from build123d import *

# Parameters (mm, degrees)
F1_DEPTH  = 873.125
F4_DEPTH  = 12.7
F5_W      = 304.8
F5_H      = 171.45
F5_R      = 17.4625
F5_W_2    = 234.95
F6_DEPTH  = 25.4
F7_W      = 101.6
F7_H      = 787.4
F7_R      = 14.2875
F8_DEPTH  = 25.4
F9_W      = 180.848
F9_H      = 241.3
F10_DEPTH = 12.7
F12_W     = 333.248
F12_H     = 409.448
F13_DEPTH = 12.7
F14_SIZE  = 168.148
F16_R     = 7.14375
F17_DEPTH = 422.149
F18_W     = 180.848
F18_H     = 241.3
F18_R     = 7.324206161
F18_R_2   = 7.2547005792
F18_R_3   = 7.130511654
F18_R_4   = 7.4581094532
F19_DEPTH = 25.4


with BuildPart() as f1:
    # F0 (on Right) → F1 (new body, symmetric)
    with BuildSketch(Plane.YZ):
        with BuildLine():
            Line((361.95, 211.074), (-361.95, 211.074))
            ThreePointArc((-361.95, 211.074), (-384.4006403027, 201.7746403027), (-393.7, 179.324))
            Line((-393.7, 179.324), (-393.7, -179.324))
            ThreePointArc((-393.7, -179.324), (-399.2796158184, -192.7943841816), (-412.75, -198.374))
            Line((-412.75, -198.374), (-520.7, -198.374))
            Line((-520.7, -198.374), (-520.7, -211.074))
            Line((-520.7, -211.074), (-412.75, -211.074))
            ThreePointArc((-412.75, -211.074), (-390.2993596973, -201.7746403027), (-381, -179.324))
            Line((-381, -179.324), (-381, 179.324))
            ThreePointArc((-381, 179.324), (-375.4203841816, 192.7943841816), (-361.95, 198.374))
            Line((-361.95, 198.374), (361.95, 198.374))
            ThreePointArc((361.95, 198.374), (375.4203841816, 192.7943841816), (381, 179.324))
            Line((381, 179.324), (381, -179.324))
            ThreePointArc((381, -179.324), (390.2993596973, -201.7746403027), (412.75, -211.074))
            Line((412.75, -211.074), (520.7, -211.074))
            Line((520.7, -211.074), (520.7, -198.374))
            Line((520.7, -198.374), (412.75, -198.374))
            ThreePointArc((412.75, -198.374), (399.2796158184, -192.7943841816), (393.7, -179.324))
            Line((393.7, -179.324), (393.7, 179.324))
            ThreePointArc((393.7, 179.324), (384.4006403027, 201.7746403027), (361.95, 211.074))
        make_face()
    extrude(amount=F1_DEPTH, both=True)

    # F5 (on face) → F6 (join)
    with BuildSketch(Plane.XY.offset(211.074)):
        with Locations((-415.925, -269.875)):
            Rectangle(F5_W, F5_H)
        with Locations((-460.375, -285.75)):
            Circle(F5_R, mode=Mode.SUBTRACT)
        with Locations((254, -269.875)):
            Rectangle(F5_W_2, F5_H)
        with Locations((263.525, -285.75)):
            Circle(F5_R, mode=Mode.SUBTRACT)
        with Locations((-415.925, 269.875)):
            Rectangle(F5_W, F5_H)
        with Locations((-460.375, 285.75)):
            Circle(F5_R, mode=Mode.SUBTRACT)
        with Locations((254, 269.875)):
            Rectangle(F5_W_2, F5_H)
        with Locations((263.525, 285.75)):
            Circle(F5_R, mode=Mode.SUBTRACT)
    extrude(amount=F6_DEPTH)

    # F7 (on face) → F8 (join)
    with BuildSketch(Plane.XY.offset(211.074)):
        with Locations((457.327, 76.2)):
            Rectangle(F7_W, F7_H)
        with Locations((460.375, -234.95)):
            Circle(F7_R, mode=Mode.SUBTRACT)
        with Locations((460.375, 234.95)):
            Circle(F7_R, mode=Mode.SUBTRACT)
        with Locations((793.623, 76.2)):
            Rectangle(F7_W, F7_H)
        with Locations((790.575, -234.95)):
            Circle(F7_R, mode=Mode.SUBTRACT)
        with Locations((790.575, 234.95)):
            Circle(F7_R, mode=Mode.SUBTRACT)
    extrude(amount=F8_DEPTH)

    # F9 (on face) → F10 (join)
    with BuildSketch(Plane.XY.offset(211.074)):
        with Locations((963.549, 0)):
            Rectangle(F9_W, F9_H)
    extrude(amount=-F10_DEPTH)



with BuildPart() as f4:
    # F3 (on offset) → F4 (new body)
    with BuildSketch(Plane.YZ.offset(720.725)):
        Polygon((361.95, 198.374), (-361.95, 198.374), (-381, 179.324), (-381, -211.074), (381, -211.074), (381, 179.324), align=None)
    extrude(amount=-F4_DEPTH)


with BuildPart() as f13:
    # F12 (on offset) → F13 (new body)
    with BuildSketch(Plane.XZ.offset(-95.25)):
        with Locations((887.349, -6.35)):
            Rectangle(F12_W, F12_H)
    extrude(amount=-F13_DEPTH)

    # F14
    f14_edges = [f13.edges().sort_by_distance(p)[0] for p in [
        (1053.973, 101.6, -211.074),
    ]]
    chamfer(f14_edges, length=F14_SIZE)


with BuildPart() as f1_1:
    add(f1.part)

    add(f4.part)  # F15 merges F4
    # F15: F13 across plane
    add(f13.part.mirror(Plane.XZ))

    # F16 (on face) → F17 (cut, through all)
    with BuildSketch(Plane.XY.offset(211.074)):
        with Locations((916.051, 63.5)):
            Circle(F16_R)
        with Locations((1017.651, 63.5)):
            Circle(F16_R)
        with Locations((1017.651, -63.5)):
            Circle(F16_R)
        with Locations((916.051, -63.5)):
            Circle(F16_R)
    extrude(amount=-F17_DEPTH, mode=Mode.SUBTRACT)


    add(f13.part)  # F19 merges F13
    # F18 (on face) → F19 (join)
    with BuildSketch(Plane.XY.offset(211.074)):
        with Locations((963.549, 0)):
            Rectangle(F18_W, F18_H)
        with Locations((916.051, -63.5)):
            Circle(F18_R, mode=Mode.SUBTRACT)
        with Locations((1017.651, -63.5)):
            Circle(F18_R_2, mode=Mode.SUBTRACT)
        with Locations((916.051, 63.5)):
            Circle(F18_R_3, mode=Mode.SUBTRACT)
        with Locations((1017.651, 63.5)):
            Circle(F18_R_4, mode=Mode.SUBTRACT)
    extrude(amount=F19_DEPTH)


solid = f1_1.part
Geometry check sheet. Reference: the model listing, model coordinates, mm. A direction names the side the tool comes from. Give positions to 0.01 mm unless a question says otherwise; leave off trailing zeros. Write each loop counter-clockwise with the first axis right and the second up, starting at its lowest first coordinate (ties: lowest second). Pieces come first, ordered by that corner, then holes. Notation, with made-up numbers: M 9,-29 L 19,-29 A27 cw 19,-11 Z; hole C -8,51 d4. An arc over 180 degrees is marked long. One line per question, with ' | ' between items.
1. Mould release check, pull along Y, two halves, no side actions. Record for faces 6 (the face through (12, 466, -211.074)), 7 (the face through (816, 233, 198.374)): released by +Y, released by -Y, zero draft, split by the parting line, or undercut.
Ans:
face 6: zero draft | face 7: undercut
2. Cross-section at C-C (y = 162). Enter the section's corners in (x, z) (3 decimals).
Ans:
outline: M -873.125,198.374 L 708.025,198.374 L 708.025,-211.074 L 720.725,-211.074 L 720.725,198.374 L 873.125,198.374 L 873.125,211.074 L 844.423,211.074 L 844.423,236.474 L 742.823,236.474 L 742.823,211.074 L 508.127,211.074 L 508.127,236.474 L 406.527,236.474 L 406.527,211.074 L -873.125,211.074 Z
3. Scan lines: line 1 along X through (y, z) = (-234, 224) (3 decimals); line 2 along Y through (x, z) = (834, -159); line 3 along X through (y, z) = (63, 205) (3 decimals). Record each from-to range of solid material in increasing order. Write a range as from..to.
Ans:
line 1: -568.325..-263.525, 136.525..371.475, 406.527..446.119, 474.631..508.127, 742.823..776.319, 804.831..844.423 | line 2: -393.7..-381, -107.95..-95.25, 95.25..107.95, 381..393.7 | line 3: -873.125..908.925, 923.177..1010.525, 1024.777..1053.973
4. Gauge pin test, flat ends, axial feed: pin 1 (4 mm diameter, centred on x = 558, y = 279, fed in from +Z); pin 2 (9 mm diameter, centred on x = 916.051, y = -63.5, fed in from -Z); pin 3 (5 mm diameter, centred on x = 286, y = -62.5, fed in from -Z); pin 4 (1.5 mm diameter, centred on y = -77, z = -4.5, fed in from -X) (3 decimals). Record the tip position at first contact, or that the pin passes through.
Ans:
pin 1: z = 211.07 | pin 2: through | pin 3: z = 198.37 | pin 4: x = 708.025
5. Cross-section at A-A (z = -3.5). Enter the section's corners in (x, y) (3 decimals), plus the area to 3 significant figures.
Ans:
outline: M -873.125,-393.7 L 873.125,-393.7 L 873.125,-381 L 720.725,-381 L 720.725,-107.95 L 1053.973,-107.95 L 1053.973,-95.25 L 720.725,-95.25 L 720.725,95.25 L 1053.973,95.25 L 1053.973,107.95 L 720.725,107.95 L 720.725,381 L 873.125,381 L 873.125,393.7 L -873.125,393.7 L -873.125,381 L 708.025,381 L 708.025,-381 L -873.125,-381 Z | area: 62,500 mm2
6. Cross-section at D-D (x = -163). Enter the section's corners in (y, z).
Ans:
outline: M -520.7,-211.07 L -412.75,-211.07 A31.75 ccw -381,-179.32 L -381,179.32 A19.05 cw -361.95,198.37 L 361.95,198.37 A19.05 cw 381,179.32 L 381,-179.32 A31.75 ccw 412.75,-211.07 L 520.7,-211.07 L 520.7,-198.37 L 412.75,-198.37 A19.05 cw 393.7,-179.32 L 393.7,179.32 A31.75 ccw 361.95,211.07 L -361.95,211.07 A31.75 ccw -393.7,179.32 L -393.7,-179.32 A19.05 cw -412.75,-198.37 L -520.7,-198.37 Z
7. Set-up check for faces 1 (the face through (885, 107.95, -3)), 2 (the face through (873.125, 379, 189)), 3 (the face through (873.125, -381, 189)), 4 (the face through (708.025, -5, -3)), 5 (the face through (264, 286, 211.074)): record each of +Z, -Z, +X, -X, +Y, -Y from which the full face is reachable in a straight line by a thin tool's end or side.
Ans:
face 1: -Z, +X | face 2: +Z, -Z, +X, +Y | face 3: +Z, -Z, +X, -Y | face 4: -Z, -X | face 5: +Z
8. Cross-section at B-B (x = -511). Enter the section's corners in (y, z), plus the area to 3 significant figures.
Ans:
outline: M -520.7,-211.07 L -412.75,-211.07 A31.75 ccw -381,-179.32 L -381,179.32 A19.05 cw -361.95,198.37 L 361.95,198.37 A19.05 cw 381,179.32 L 381,-179.32 A31.75 ccw 412.75,-211.07 L 520.7,-211.07 L 520.7,-198.37 L 412.75,-198.37 A19.05 cw 393.7,-179.32 L 393.7,179.32 A31.75 ccw 361.95,211.07 L 355.6,211.07 L 355.6,236.47 L 184.15,236.47 L 184.15,211.07 L -184.15,211.07 L -184.15,236.47 L -355.6,236.47 L -355.6,211.07 L -361.95,211.07 A31.75 ccw -393.7,179.32 L -393.7,-179.32 A19.05 cw -412.75,-198.37 L -520.7,-198.37 Z | area: 31,800 mm2
